Autodesk Inventor part; units mm, degrees
ref_plane "Work Plane1" through (0, 12.7, 0) normal (0, 1, 0) x (1, 0, 0)
ref_plane "Work Plane2" through (0, 88.9, 0) normal (0, 1, 0) x (1, 0, 0)
ref_plane "YZ Plane" through (0, 0, 0) normal (1, 0, 0) x (0, 1, 0)
ref_plane "Work Plane1" through (0, 12.7, 0) normal (0, 1, 0) x (1, 0, 0)
sketch "Sketch3" plane through (0, 12.7, 0) normal (0, 1, 0) x (1, 0, 0)
  line L0 (-144.4503, 24.8067) -> (-122.2253, 63.3015)
  line L1 (-126.6247, 70.9215) -> (-122.2253, 63.3015)
  line L2 (-122.2253, 63.3015) -> (-81.5853, 63.3015)
  line L3 (-126.6247, 70.9215) -> (-151.3441, 28.1063)
  line L4 (-133.3378, 44.0541) -> (-139.9369, 47.8641)
  line L5 (-151.3441, 28.1063) -> (-142.5453, 28.1063)
  line L6 (-126.6247, 70.9215) -> (-77.1859, 70.9215)
  line L7 (-81.5853, 63.3015) -> (-77.1859, 70.9215)
  line L8 (-151.3441, 28.1063) -> (-155.6743, 30.6063)
  line L9 (-151.3441, 28.1063) -> (-146.3441, 28.1063) construction
  line L10 (-155.6743, 30.6063) -> (-129.5115, 75.9215)
  line L11 (-130.9549, 73.4215) -> (-126.6247, 70.9215)
  line L12 (-126.6247, 70.9215) -> (-129.5115, 75.9215)
  line L13 (-126.6247, 70.9215) -> (-119.7825, 70.9215) construction
  line L14 (-80.0727, 75.9215) -> (-77.1859, 70.9215)
  line L15 (-129.5115, 75.9215) -> (-80.0727, 75.9215)
  line L16 (-91.4611, 75.9215) -> (-90.9796, 70.9215)
  point P0 (-77.3883, 70.9215)
  dimension "d84" = 44.45
  dimension "d85" = 120
  dimension "d86" = 7.62
  dimension "d105" = 120
  dimension "d133" = 40.64
  dimension "d134" = 120
  dimension "d135" = 7.62
  dimension "d160" = 90
  dimension "d163" = 5
  dimension "d164" = 150
  dimension "d166" = 5
  dimension "d168" = 120
ref_plane "Work Plane2" through (0, 88.9, 0) normal (0, 1, 0) x (1, 0, 0)
extrude "Extrusion16" add sketch "Sketch3" along normal blind 12.7 contours L5 L3 L4 L0 | L4 L3 L1 L0 | L1 L6 L7 L2
sketch "Sketch8" plane through (0, 12.7, 0) normal (0, -1, 0) x (1, 0, 0)
  line L0 (-81.5853, -63.3015) -> (-77.1859, -70.9215)
  line L1 (-77.1859, -70.9215) -> (-73.0826, -70.9215) construction
  line L2 (-77.1859, -70.9215) -> (-77.1859, -110.9215)
  line L3 (-77.1859, -70.9215) -> (-126.6247, -70.9215)
  line L4 (-77.1859, -70.9215) -> (-37.1859, -70.9215) construction
  line L5 (-77.1859, -110.9215) -> (-93.1859, -110.9215)
  line L6 (-93.1859, -110.9215) -> (-93.1859, -70.9215)
  point P0 (0, 0)
  dimension "d137" = 40
  dimension "d138" = 90
  dimension "d139" = 16
extrude "Extrusion18" add sketch "Sketch8" against normal blind 12.7
sketch "Sketch9" plane through (0, 25.4, 0) normal (0, 1, 0) x (1, 0, 0)
  line L0 (-93.1859, 110.9215) -> (-77.1859, 110.9215)
  line L1 (-77.1859, 110.9215) -> (-80.1859, 110.9215)
  line L2 (-93.1859, 110.9215) -> (-90.1859, 110.9215)
  line L3 (-80.1859, 110.9215) -> (-80.1859, 72.2521)
  line L4 (-80.1859, 110.9215) -> (-41.5165, 110.9215) construction
  line L5 (-90.1859, 110.9215) -> (-90.1859, 72.2521)
  line L6 (-90.1859, 72.2521) -> (-80.1859, 72.2521)
  point P0 (0, 0)
  dimension "d142" = 3
  dimension "d143" = 3
  dimension "d144" = 90
extrude "Extrusion20" [suppressed]
extrude "Extrusion21" cut sketch "Sketch9" against normal blind 4
extrude "Extrusion22" add sketch "Sketch3" along normal blind 12.7 contours L8 L10 L11 L3 | L12 L15 L16 L6 | L11 L10 L12
properties part number "HorizGrabberMoving"
Geometry: final body of the model. Coordinates: model frame, mm. A direction names the side the tool comes from. Give positions to 0.01 mm unless a question says otherwise; leave off trailing zeros. Loops run counter-clockwise (first coordinate to the right, second up) from the corner with the lowest first, then second, coordinate; pieces in that order, holes last. Notation, with made-up numbers: (55.5, 61.25) - (106.5, 61.25) arc R21 cw to (106.5, 78.25) - close; hole circle Ø9 at (23, 16). An arc over 180 degrees is marked (long way). Answer as CSV lines item,"result". Start each with the question number.
(1) Ray query, line 1 along X through (y, z) = (23.5, -105); line 2 along Z through (x, y) = (-93.5, 24.75); line 3 along X through (y, z) = (19, -105.5). Return the intervals inside material, ascending. Write a range as [from, to].
(2) Reachability of faces 4 (the face through (-77.186, 19, -91)), 5 (the face through (-120, 25.4, -66)), 6 (the face through (-85, 23, -72.252)), 7 (the face through (-102, 19, -63.302)), 8 (the face through (-93.186, 19, -94)) from +Z, -Z, +X, -X, +Y, -Y: full face, straight path, thin tool, end or side. Return the list, or none.
(3) Pin query (flat end, axial travel): P1, Ø4, axis at y = 21.5, z = -83, coming from the -X side; P2, Ø4, axis at x = -112, y = 20, coming from the -Z side; P3, Ø11, axis at x = -87, z = -88.5, coming from the +Y side; P4, Ø4, axis at x = -105.5, y = 18, coming from the +Z side. Return the tip coordinate at first contact, or that it passes through.
(4) Section query D-D (y = 17.25). Output: boundary loops of the cut face in (x, z), and give its area (3 significant figures).
(5) Section query C-C (x = -100). Output: boundary loops of the cut face in (y, z).
(6) Mould query, pull axis X, two halves, no side actions, for faces 1 (the face through (-132.528, 18.961, -45.458)), 2 (the face through (-85, 21.4, -92)), 3 (the face through (-112, 19, -75.922)). Classes: +X half, -X half, draft (parallel to the pull), parting line (faces both ways), or undercut.
(7) Section query A-A (z = -80). Output: boundary loops of the cut face in (x, y).
(8) Section query B-B (y = 23.5). Output: boundary loops of the cut face in (x, z), and give its area (3 significant figures).
Worked answers:
1,line 1,"x = [-93.19, -90.19], [-80.19, -77.19]"
1,line 2,"z = [-75.92, -63.3]"
1,line 3,"x = [-93.19, -77.19]"
2,face 4,"+Z, -Z, +X, +Y, -Y"
2,face 5,"+Z, -Z, +X, -X, +Y"
2,face 6,"-Z, +Y"
2,face 7,"+Z, +X, +Y, -Y"
2,face 8,"-Z, -X, +Y, -Y"
3,P1,"stops at x = -93.19"
3,P2,"stops at z = -75.92"
3,P3,"stops at y = 25.4"
3,P4,"stops at z = -63.3"
4,outline,"(-155.67, -30.61) - (-129.51, -75.92) - (-93.19, -75.92) - (-93.19, -110.92) - (-77.19, -110.92) - (-77.19, -70.92) - (-81.59, -63.3) - (-122.23, -63.3) - (-142.55, -28.11) - (-151.34, -28.11) - close"
4,area,"1,760 mm^2"
5,outline,"(12.7, -75.92) - (25.4, -75.92) - (25.4, -63.3) - (12.7, -63.3) - close"
6,face 1,"+X half"
6,face 2,"undercut"
6,face 3,"draft"
7,outline,"(-93.19, 12.7) - (-77.19, 12.7) - (-77.19, 25.4) - (-80.19, 25.4) - (-80.19, 21.4) - (-90.19, 21.4) - (-90.19, 25.4) - (-93.19, 25.4) - close"
8,outline,"(-155.67, -30.61) - (-129.51, -75.92) - (-93.19, -75.92) - (-93.19, -110.92) - (-90.19, -110.92) - (-90.19, -72.25) - (-80.19, -72.25) - (-80.19, -110.92) - (-77.19, -110.92) - (-77.19, -70.92) - (-81.59, -63.3) - (-122.23, -63.3) - (-142.55, -28.11) - (-151.34, -28.11) - close"
8,area,"1,370 mm^2"
